Geometry check sheet. Reference: drawing and pictorial views, mm from the part's lowest x, y, z. Give positions to 0.01 mm unless a question says otherwise; leave off trailing zeros. Write each loop counter-clockwise with the first axis right and the second up, starting at its lowest first coordinate (ties: lowest second). Pieces come first, ordered by that corner, then holes. Notation, with made-up numbers: (75, -30.5) - (122, -30.5) arc R19 cw to (122, 0.5) - close; hole circle Ø2 at (45, -27.75). An arc over 180 degrees is marked (long way). Write item = value, one per line. Start each with the question number.
(1) Section check C-C, the plane z = 49. Enter the section's corners in (x, y).
(2) Section check A-A, the plane x = 21.5. Enter the section's corners in (y, z).
(3) Section check D-D, the plane z = 7.5. Enter the section's corners in (x, y).
(4) Thickness scan on L1, parallel to X at y = 1.95, z = 24; L2, parallel to Z at x = 35, y = 2.1; L3, parallel to Z at x = 38.5, y = 2.2. Record the ranges inside material, lowest first.
(5) Section check B-B, the plane y = 1.55. Enter the section's corners in (x, z).
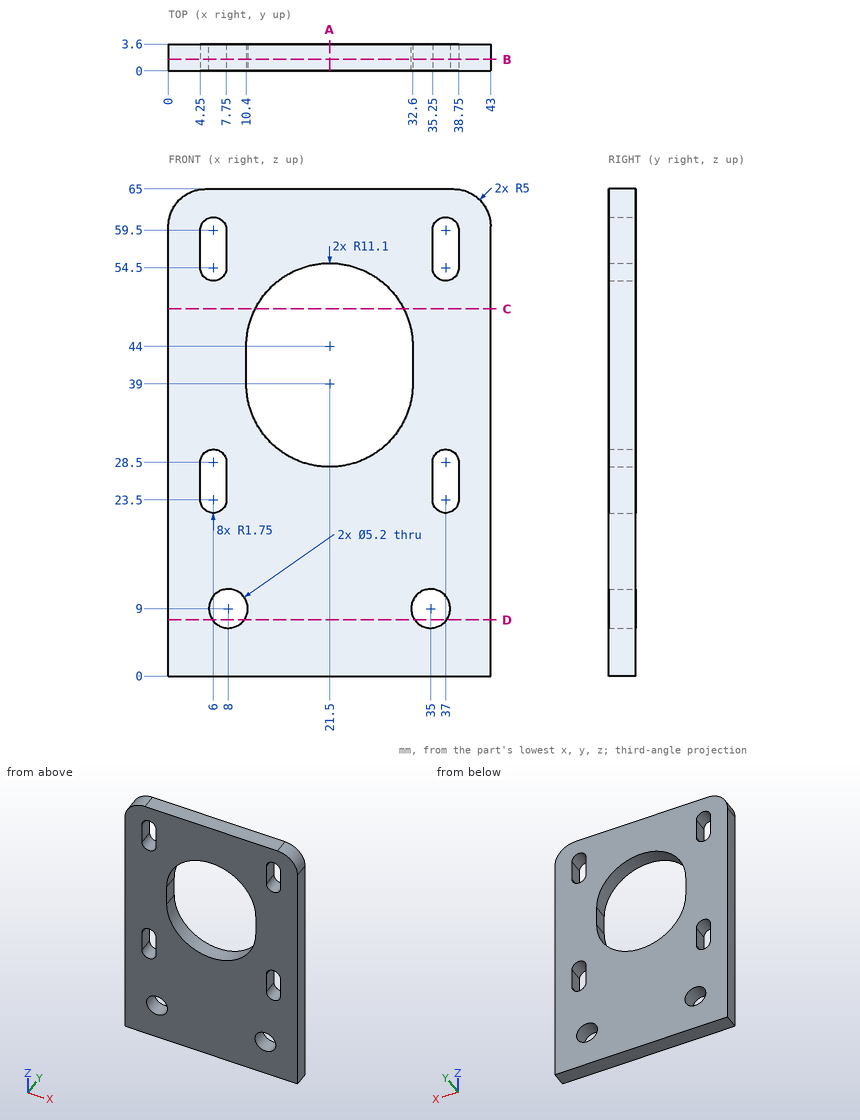
Model answer:
q1.outline = (0, 0) - (11.59, 0) - (11.59, 3.6) - (0, 3.6) - close; (31.41, 0) - (43, 0) - (43, 3.6) - (31.41, 3.6) - close
q2.outline = (0, 0) - (3.6, 0) - (3.6, 27.9) - (0, 27.9) - close; (0, 55.1) - (3.6, 55.1) - (3.6, 65) - (0, 65) - close
q3.outline = (0, 0) - (5.88, 0) - (5.88, 3.6) - (0, 3.6) - close; (10.12, 0) - (32.88, 0) - (32.88, 3.6) - (10.12, 3.6) - close; (37.12, 0) - (43, 0) - (43, 3.6) - (37.12, 3.6) - close
q4.L1 = 0 to 4.25, 7.75 to 35.25, 38.75 to 43
q4.L2 = 0 to 6.4, 11.6 to 65
q4.L3 = 0 to 22.6, 29.4 to 53.6, 60.4 to 64.97
q5.outline = (0, 0) - (43, 0) - (43, 60) arc R5 ccw to (38, 65) - (5, 65) arc R5 ccw to (0, 60) - close; hole (4.25, 23.5) arc R1.75 ccw to (7.75, 23.5) - (7.75, 28.5) arc R1.75 ccw to (4.25, 28.5) - close; hole (4.25, 54.5) arc R1.75 ccw to (7.75, 54.5) - (7.75, 59.5) arc R1.75 ccw to (4.25, 59.5) - close; hole circle Ø5.2 at (8, 9); hole (10.4, 39) arc R11.1 ccw to (32.6, 39) - (32.6, 44) arc R11.1 ccw to (10.4, 44) - close; hole circle Ø5.2 at (35, 9); hole (35.25, 23.5) arc R1.75 ccw to (38.75, 23.5) - (38.75, 28.5) arc R1.75 ccw to (35.25, 28.5) - close; hole (35.25, 54.5) arc R1.75 ccw to (38.75, 54.5) - (38.75, 59.5) arc R1.75 ccw to (35.25, 59.5) - close
